Source: CAD feature listing. Evaluate the final solid. Frame: model axes, mm. A direction names the side the tool comes from. Coordinates: 2 decimals unless noted, no trailing zeros. Loops run counter-clockwise (first coordinate to the right, second up) from the corner with the lowest first, then second, coordinate; pieces in that order, holes last. Notation, with made-up numbers: (-19, 11) - (21, 11) arc R18 cw to (21, 19) - close; hole circle Ø5 at (-24.5, 86). An arc over 180 degrees is marked (long way). Use one line per item in the form item = value. Start each with the question number.
from build123d import *

# Parameters (mm, degrees)
BOSS_EXTRUDE1_DEPTH = 15
BOSS_EXTRUDE2_DEPTH = 15


with BuildPart() as part:
    # Sketch1 → Boss-Extrude1 (new body)
    with BuildSketch(Plane.XY):
        Polygon((0, 25), (0, 0), (25, 0), align=None)
    extrude(amount=BOSS_EXTRUDE1_DEPTH)

    # Sketch2 → Boss-Extrude2 (add)
    with BuildSketch(Plane(origin=(0, 0, 0), x_dir=(-1, 0, 0), z_dir=(0, 0, -1))):
        Polygon((-25, 0), (-25, 25), (0, 0), align=None)
    extrude(amount=BOSS_EXTRUDE2_DEPTH)


solid = part.part
(1) Cut plane B-B, the plane y = 11.25. Output: boundary loops of the cut face in (x, z), plus the area to 4 significant figures.
(2) Contact query for flat-ended pins moving along their axis: pin 1 (2 mm diameter, centred on x = 16, z = -3.5, fed in from +Y); pin 2 (4 mm diameter, centred on x = 17, y = 15.5, fed in from +Z); pin 3 (12 mm diameter, centred on y = 9, z = -10, fed in from -X); pin 4 (14 mm diameter, centred on x = 8.5, y = 17.5, fed in from -Z). Output: stop coordinate, or through.
(3) Cut plane A-A, the plane y = 14.75. Output: boundary loops of the cut face in (x, z), plus the area to 4 significant figures.
(4) Access query for faces 1 (the face through (18, 7, -15)), 2 (the face through (5, 13, 0)), 3 (the face through (20, 13, 0)). Directions: +Z, -Z, +X, -X, +Y, -Y. A direction counts if a zero-diameter tool reaches every point of the face in a straight line with its end or side. Return the directions, or none.
(5) Material intervals for line 1 (Y direction, x = 12.5, z = 14); line 2 (Z direction, x = 1.75, y = 13); line 3 (Z direction, x = 14.5, y = 12.25), sorted ascending.
(6) Cut plane C-C, the plane x = 16.5. Output: boundary loops of the cut face in (y, z), plus the area to 3 significant figures.
(7) Cut plane D-D, the plane y = 20.75. Output: boundary loops of the cut face in (x, z).
Recorded:
q1.outline = (0, 0) - (11.25, 0) - (11.25, -15) - (25, -15) - (25, 0) - (13.75, 0) - (13.75, 15) - (0, 15) - close
q1.area = 412.5 mm²
q2.pin_1 = 17
q2.pin_2 = 0
q2.pin_3 = 3
q2.pin_4 = -15
q3.outline = (0, 0) - (10.25, 0) - (10.25, 15) - (0, 15) - close; (14.75, -15) - (25, -15) - (25, 0) - (14.75, 0) - close
q3.area = 307.5 mm²
q4.face_1 = -Z, +X, -X, +Y, -Y
q4.face_2 = -Z, -X, +Y
q4.face_3 = +Z, +X, +Y
q5.line_1 = 0 to 12.5
q5.line_2 = 0 to 15
q5.line_3 = -15 to 0
q6.outline = (0, -15) - (16.5, -15) - (16.5, 0) - (8.5, 0) - (8.5, 15) - (0, 15) - close
q6.area = 375 mm²
q7.outline = (0, 0) - (4.25, 0) - (4.25, 15) - (0, 15) - close; (20.75, -15) - (25, -15) - (25, 0) - (20.75, 0) - close
